Input: part model. Units: mm. Frame: model coordinates. A direction names the side the tool comes from. Round coordinates to 2 decimals unless told otherwise and drop trailing zeros. Loops run counter-clockwise (first coordinate to the right, second up) from the corner with the lowest first, then second, coordinate; pieces in that order, holes last.
(1) Cut plane C-C, the plane z = 17. Output: boundary loops of the cut face in (x, y), and give its area (3 significant figures).
(2) Access query for faces 1 (the face through (-54.675, 22, 1)), 2 (the face through (-14, 22, 3)), 3 (the face through (-40.562, 34.236, 46.461)), 4 (the face through (-56, 22, 3)). Directions: +Z, -Z, +X, -X, +Y, -Y. A direction counts if a zero-diameter tool reaches every point of the face in a straight line with its end or side. Return the directions, or none.
(3) First-contact query: pin 1 Ø3.5 at (x, y) = (29.5, 24) entering from -Z; pin 2 Ø1.8 at (x, z) = (-39.67, 46) entering from +Y; pin 3 Ø2 at (x, y) = (5, 20) entering from +Z. Flat tips, straight axial feed; report the tip coordinate or a pass-through.
(4) Draft query along Z for faces 5 (the face through (27.325, 22, 1)), 6 (the face through (12.025, 34.236, 45.046)), 7 (the face through (-14, 22, 0)). Return one class per face: released by +Z, released by -Z, zero draft, split by the parting line, or undercut.
(5) Line query: line 1 (X direction, y = 34.9, z = 46); line 2 (Y direction, x = -11, z = 41); line 3 (X direction, y = 27, z = 27). Output: solid intervals per line, ascending.
(6) Cut plane B-B, the plane y = 13. Output: boundary loops of the cut face in (x, z), and give its area (3 significant figures).
(7) Cut plane D-D, the plane x = 21.5. Output: boundary loops of the cut face in (y, z).
(8) Cut plane A-A, the plane z = 46. Output: boundary loops of the cut face in (x, y), and give its area (3 significant figures).
from build123d import *

# Parameters (mm, degrees)
SKETCH_1_W          = 88
SKETCH_1_H          = 28
EXTRUDE_1_DEPTH     = 48
SHELL_1_T           = -3
SKETCH_2_R          = 1
CUT_EXTRUDE_1_DEPTH = 3
SKETCH_5_W          = 15
SKETCH_5_H          = 22
CUT_EXTRUDE_4_DEPTH = 107.412344412
SKETCH_6_W          = 15
SKETCH_6_H          = 22
CUT_EXTRUDE_5_DEPTH = 15


with BuildPart() as part:
    # 草圖1 → 填料-伸長1 (new body)
    with BuildSketch(Plane.XY):
        with Locations((-13.67483766, 21.715361446)):
            Rectangle(SKETCH_1_W, SKETCH_1_H)
    extrude(amount=EXTRUDE_1_DEPTH)

    # 薄殼1
    shell_1_openings = [part.faces().sort_by_distance(p)[0] for p in [
        (-13.67483766, 21.715361446, 48),
    ]]
    offset(amount=SHELL_1_T, openings=shell_1_openings, kind=Kind.INTERSECTION)

    # 草圖2 → 除料-伸長1 (cut)
    with BuildSketch(Plane(origin=(0, 35.715361446, 0), x_dir=(1, 0, 0), z_dir=(0, 1, 0))):
        with Locations(Location((-31.67483766, -46, 0), (0, 0, 270))):
            Circle(SKETCH_2_R)
        with Locations(Location((-39.67483766, -46, 0), (0, 0, 270))):
            Circle(SKETCH_2_R)
        with Locations(Location((12.32516234, -46, 0), (0, 0, 90))):
            Circle(SKETCH_2_R)
        with Locations(Location((4.32516234, -46, 0), (0, 0, 90))):
            Circle(SKETCH_2_R)
    extrude(amount=-CUT_EXTRUDE_1_DEPTH, mode=Mode.SUBTRACT)

    # 草圖5 → 除料-伸長4 (cut, through all)
    with BuildSketch(Plane.ZY.offset(57.67483766)):
        with Locations((10.5, 21.715361446)):
            Rectangle(SKETCH_5_W, SKETCH_5_H)
    extrude(amount=-CUT_EXTRUDE_4_DEPTH, mode=Mode.SUBTRACT)

    # 草圖6 → 除料-伸長5 (cut)
    with BuildSketch(Plane(origin=(0, 0, 0), x_dir=(-1, 0, 0), z_dir=(0, 0, -1))):
        with Locations((-19.82516234, 21.715361446)):
            Rectangle(SKETCH_6_W, SKETCH_6_H)
        with Locations((47.17483766, 21.715361446)):
            Rectangle(SKETCH_6_W, SKETCH_6_H)
    extrude(amount=-CUT_EXTRUDE_5_DEPTH, mode=Mode.SUBTRACT)


solid = part.part
Reported:
1. outline: (-57.67, 7.72) - (30.33, 7.72) - (30.33, 10.72) - (-57.67, 10.72) - close; (-57.67, 32.72) - (30.33, 32.72) - (30.33, 35.72) - (-57.67, 35.72) - close
1. area: 528 mm2
2. face 1: +Z, -Z
2. face 2: +Z, +X, -X
2. face 3: +Y
2. face 4: +X, -X
3. pin 1: stops at z = 0
3. pin 2: stops at y = 10.72
3. pin 3: stops at z = 3
4. face 5: zero draft
4. face 6: undercut
4. face 7: released by -Z
5. line 1: x = -57.67 to -40.67, -38.67 to -32.67, -30.67 to 3.33, 5.33 to 11.33, 13.33 to 30.33
5. line 2: y = 7.72 to 10.72, 32.72 to 35.72
5. line 3: x = -57.67 to -54.67, 27.33 to 30.33
6. outline: (-57.67, 0) - (-54.67, 0) - (-54.67, 3) - (-57.67, 3) - close; (-57.67, 18) - (-54.67, 18) - (-54.67, 48) - (-57.67, 48) - close; (-39.67, 0) - (12.33, 0) - (12.33, 3) - (-39.67, 3) - close; (27.33, 0) - (30.33, 0) - (30.33, 3) - (27.33, 3) - close; (27.33, 18) - (30.33, 18) - (30.33, 48) - (27.33, 48) - close
6. area: 354 mm2
7. outline: (7.72, 0) - (10.72, 0) - (10.72, 48) - (7.72, 48) - close; (32.72, 0) - (35.72, 0) - (35.72, 48) - (32.72, 48) - close
8. outline: (-57.67, 7.72) - (30.33, 7.72) - (30.33, 35.72) - (13.33, 35.72) - (13.33, 32.72) - (27.33, 32.72) - (27.33, 10.72) - (-54.67, 10.72) - (-54.67, 32.72) - (-40.67, 32.72) - (-40.67, 35.72) - (-57.67, 35.72) - close; (-38.67, 32.72) - (-32.67, 32.72) - (-32.67, 35.72) - (-38.67, 35.72) - close; (-30.67, 32.72) - (3.33, 32.72) - (3.33, 35.72) - (-30.67, 35.72) - close; (5.33, 32.72) - (11.33, 32.72) - (11.33, 35.72) - (5.33, 35.72) - close
8. area: 636 mm2
